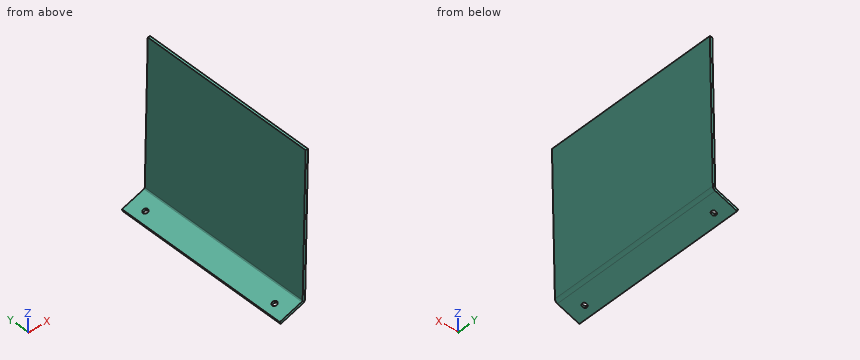
from build123d import *

# Parameters (mm, degrees)
BASE_FLANGE1_DEPTH          = 110
F_3_0MM_PRESS_DOWEL_HOLE1_D = 3


# Sheet-metal steps are written as plain solids
with BuildPart() as part:
    # Sketch1 → Base-Flange1 (new body)
    with BuildSketch(Plane(origin=(0, 0, 0), x_dir=(1, 0, 0), z_dir=(0, 1, 0))):
        with BuildLine():
            Line((0, 0), (-1.855570085, 89.464986247))
            ThreePointArc((-1.855570085, 89.464986247), (-1.99751505, 89.884629471), (-2.354487023, 90.146964789))
            Line((-2.354487023, 90.146964789), (-16.065007208, 94.817561297))
            Line((-16.065007208, 94.817561297), (-15.5813159, 96.237435489))
            Line((-15.5813159, 96.237435489), (-1.870795715, 91.56683898))
            ThreePointArc((-1.870795715, 91.56683898), (-0.786891948, 90.770288381), (-0.355892615, 89.496090669))
            Line((-0.355892615, 89.496090669), (1.49967747, 0.031104422))
            Line((1.49967747, 0.031104422), (0, 0))
        make_face()
    extrude(amount=BASE_FLANGE1_DEPTH)

    # Ø3.0mm Press Dowel Hole1 (through all)
    with Locations(Plane(origin=(27.754960473, 0, -81.474592183), x_dir=(-0.9465827940969574, 0, -0.32246087192029516), z_dir=(0.32246087192029516, 0, -0.9465827940969574))):
        with Locations((39.781812899, 10), (39.781812899, 100)):
            Hole(F_3_0MM_PRESS_DOWEL_HOLE1_D / 2)


solid = part.part
Work out the finished part from the listing and answer in its coordinate system (mm). Round coordinates to 2 decimals unless told otherwise and drop trailing zeros. Order: outer loops, then holes, each group sorted by start corner. A loop starts at its lowest first (then second) coordinate and runs counter-clockwise, first axis right, second up. Notation, with made-up numbers: M 87,64.25 L 133,64.25 A26 cw 133,87.25 Z; hole C 84,-32 d4. An arc over 180 degrees is marked long. Put each result on its own line as item: value. Start each with the question number.
Q1. Section B-B, the plane z = -17.5 is taken. Write down the section's boundary in (x, y), and give its area (3 significant figures).
Q2. Flat-ended cylindrical pins translate along their axes: pin 1 (1.5 mm diameter, centred on y = 36.5, z = -68, fed in from -X); pin 2 (2 mm diameter, centred on y = 80.5, z = -55.5, fed in from +X); pin 3 (10 mm diameter, centred on y = 76.5, z = -65, fed in from -X). Find the tip coordinate at first contact, or state that the pin passes through.
Q3. Section A-A, the plane y = 77 is taken. Write down the section's boundary in (x, z) (3 decimals), and give its area (3 significant figures).
Q4. Straight lines are drawn through the part: L1, parallel to Z at x = -5, y = 33; L2, parallel to X at y = 42, z = -24; L3, parallel to X at y = 11, z = -81. For each, find the intervals that lie inside material, in ascending order. Write a range as [from, to].
Q5. Section C-C, the plane x = -13.25 is taken. Write down the section's boundary in (y, z).
Findings below:
1. outline: M -0.36,0 L 1.14,0 L 1.14,110 L -0.36,110 Z
1. area: 165 mm^2
2. pin 1: stops at x = -1.43
2. pin 2: stops at x = 0.37
2. pin 3: stops at x = -1.45
3. outline: M -16.065,-94.818 L -15.581,-96.237 L -1.871,-91.567 A2.237 ccw -0.356,-89.496 L 1.5,-0.031 L 0,0 L -1.856,-89.465 A0.737 cw -2.354,-90.147 Z
3. area: 159 mm^2
4. L1: z = [-92.63, -91.05]
4. L2: x = [-0.5, 1]
4. L3: x = [-1.68, -0.18]
5. outline: M 0,-95.44 L 110,-95.44 L 110,-93.86 L 0,-93.86 Z
